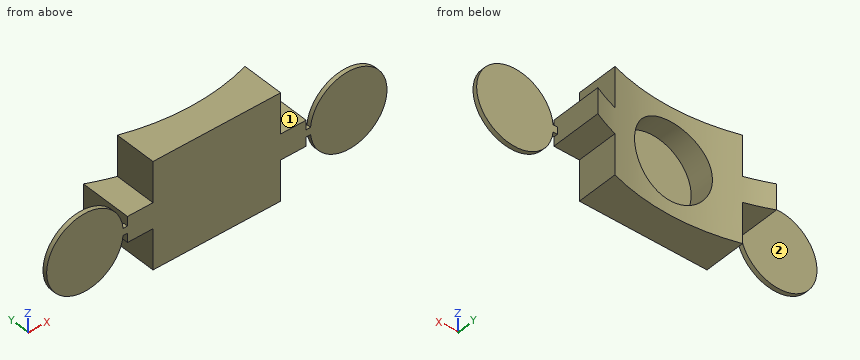
```python
from build123d import *

# Parameters (mm, degrees)
F1_DEPTH  = 12.5
F3_DEPTH  = 25
F4_R      = 9.15
F5_DEPTH  = 55
F6_R      = 9.05
F7_DEPTH  = 52.5
F9_DEPTH  = 3
F11_DEPTH = 57.501
F13_DEPTH = 1


with BuildPart() as f1:
    # F0 (on Top) → F1 (new body, symmetric)
    with BuildSketch(Plane.XY):
        with BuildLine():
            ThreePointArc((50, 0), (0, -50), (-50, 0))
            Line((-50, 0), (-55, 0))
            ThreePointArc((-55, 0), (0, -55), (55, 0))
            Line((55, 0), (50, 0))
        make_face()
    extrude(amount=F1_DEPTH, both=True)

    # F2 (on face) → F3 (join)
    with BuildSketch(Plane.XY.offset(12.5)):
        with BuildLine():
            ThreePointArc((55, 0), (0, -55), (-55, 0))
            Line((-55, 0), (-55, -57.5))
            Line((-55, -57.5), (0, -57.5))
            Line((0, -57.5), (55, -57.5))
            Line((55, -57.5), (55, 0))
        make_face()
    extrude(amount=-F3_DEPTH)

    # F4 (on Front) → F5 (cut)
    with BuildSketch(Plane.XZ):
        Circle(F4_R)
    extrude(amount=F5_DEPTH, mode=Mode.SUBTRACT)

    # F6 (on Right) → F7 (cut, symmetric)
    with BuildSketch(Plane.YZ):
        with Locations((-11, 0)):
            Circle(F6_R)
    extrude(amount=F7_DEPTH, both=True, mode=Mode.SUBTRACT)

    # F8 (on face) → F9 (join)
    with BuildSketch(Plane.XZ.offset(57.5)):
        with BuildLine():
            Line((55, -1.825145), (56.187007, -1.825145))
            ThreePointArc((56.187007, -1.825145), (73.996764, 0.241309), (56.101841, 1.350101))
            Line((56.101841, 1.350101), (55, 1.350101))
            Line((55, 1.350101), (55, -1.825145))
        make_face()
        with BuildLine():
            Line((-55, 0.589209), (-56.019308, 0.589209))
            ThreePointArc((-56.019308, 0.589209), (-73.999691, -0.074534), (-56.010781, -0.440385))
            Line((-56.010781, -0.440385), (-55, -0.440385))
            Line((-55, -0.440385), (-55, 0.589209))
        make_face()
        with BuildLine():
            Line((26.665892, -12.5), (26.665892, -13.538735))
            ThreePointArc((26.665892, -13.538735), (27.491135, -31.499996), (28.35176, -13.540396))
            Line((28.35176, -13.540396), (28.35176, -12.5))
            Line((28.35176, -12.5), (26.665892, -12.5))
        make_face()
        with BuildLine():
            Line((-28.294771, -12.5), (-28.294771, -13.535161))
            ThreePointArc((-28.294771, -13.535161), (-27.521055, -31.499975), (-26.663293, -13.538978))
            Line((-26.663293, -13.538978), (-26.663293, -12.5))
            Line((-26.663293, -12.5), (-28.294771, -12.5))
        make_face()
        with BuildLine():
            Line((-26.327094, 12.5), (-26.327094, 13.576756))
            ThreePointArc((-26.327094, 13.576756), (-27.667739, 31.498437), (-28.339533, 13.539242))
            Line((-28.339533, 13.539242), (-28.339533, 12.5))
            Line((-28.339533, 12.5), (-26.327094, 12.5))
        make_face()
        with BuildLine():
            Line((28.639116, 12.5), (28.639116, 13.572379))
            ThreePointArc((28.639116, 13.572379), (27.368028, 31.499032), (26.623167, 13.542815))
            Line((26.623167, 13.542815), (26.623167, 12.5))
            Line((26.623167, 12.5), (28.639116, 12.5))
        make_face()
    extrude(amount=-F9_DEPTH)

    # F10 (on face) → F11 (cut, through all)
    with BuildSketch(Plane.XZ.offset(57.5)):
        Polygon((-15, 3), (-15, 12.5), (-15, 43.200534), (-80.149591, 43.200534), (-80.149591, -41.894257), (-15, -41.894257), (-15, -12.5), (-15, -3), (-21, -3), (-21, 0), (-21, 3), align=None)
        Polygon((15, 42.100117), (15, 12.5), (15, 3), (21, 3), (21, 0), (21, -3), (15, -3), (15, -12.5), (15, -47.119375), (79.776369, -47.119375), (79.776369, 42.100117), align=None)
    extrude(amount=-F11_DEPTH, mode=Mode.SUBTRACT)

    # F12 (on face) → F13 (join)
    with BuildSketch(Plane.XZ.offset(57.5)):
        with BuildLine():
            Line((-21, 0.785101), (-22.034309, 0.785101))
            ThreePointArc((-22.034309, 0.785101), (-39.999944, 0.031742), (-22.04007, -0.848323))
            Line((-22.04007, -0.848323), (-21, -0.848323))
            Line((-21, -0.848323), (-21, 0.785101))
        make_face()
        with BuildLine():
            Line((21, -0.86237), (22.041411, -0.86237))
            ThreePointArc((22.041411, -0.86237), (39.99991, 0.040222), (22.034061, 0.782262))
            Line((22.034061, 0.782262), (21, 0.782262))
            Line((21, 0.782262), (21, -0.86237))
        make_face()
    extrude(amount=-F13_DEPTH)


solid = f1.part
```
Can you work these out from the model? Positions are in its coordinate system, mm. Face numbers are marked on the shaded views. A direction names the side the tool comes from. Round coordinates to 2 decimals unless told otherwise and drop trailing zeros. Order: outer loops, then holes, each group sorted by start corner. A loop starts at its lowest first (then second) coordinate and runs counter-clockwise, first axis right, second up.
(1) If we section it at C-C (y = -47): Please give me the cut outline in (x, z).
Results are:
outline: (-21, -3) - (-17.06, -3) - (-17.06, 3) - (-21, 3) - close; (17.06, -3) - (21, -3) - (21, 3) - (17.06, 3) - close
(2) On a 3-axis mill with a long thin cutter (end or side, diameter ignored), from which of +Z, -Z, +X, -X, +Y, -Y can I reach the whole of each face in a straight line? I mean the marked faces 1 and 2. Say none if no direction works.
Results are:
face 1: +Z, +Y, -Y
face 2: +Z, -Z, -X, +Y
(3) If we section it at B-B (y = -53.5): Please give me the cut outline in (x, z).
Results are:
outline: (-21, -3) - (-15, -3) - (-15, -12.5) - (15, -12.5) - (15, -3) - (21, -3) - (21, 3) - (15, 3) - (15, 12.5) - (-15, 12.5) - (-15, 3) - (-21, 3) - close; hole circle Ø18.3 at (0, 0)
(4) If we section it at A-A (z = 7.25): Please give me the cut outline in (x, y), plus the area to 3 significant figures.
Results are:
outline: (-36.33, -57.5) - (-25.67, -57.5) - (-25.67, -56.5) - (-36.33, -56.5) - close; (-15, -57.5) - (15, -57.5) - (15, -47.7) arc R50 cw to (5.58, -49.69) - (5.58, -55) - (-5.58, -55) - (-5.58, -49.69) arc R50 cw to (-15, -47.7) - close; (25.67, -57.5) - (36.33, -57.5) - (36.33, -56.5) - (25.67, -56.5) - close
area: 212 mm2
(5) I'm going to push flat-ended pins straight in: pin 1 (1 mm diameter, centred on x = 32, z = 8, fed in from +Y); pin 2 (1.8 mm diameter, centred on x = 17, y = -53.5, fed in from +Z); pin 3 (5 mm diameter, centred on y = -51.5, z = -7, fed in from -X). Where does each tip first touch, or does it pass through?
Results are:
pin 1: stops at y = -56.5
pin 2: stops at z = 3
pin 3: stops at x = -15
(6) If we section it at D-D (x = 0): Please give me the cut outline in (y, z).
Results are:
outline: (-57.5, -12.5) - (-50, -12.5) - (-50, -9.15) - (-55, -9.15) - (-55, 9.15) - (-50, 9.15) - (-50, 12.5) - (-57.5, 12.5) - close
(7) If I drill on L1, parallel to X at y = -52.9, z = 0; L2, parallel to Z at x = 0, y = -51.1; L3, parallel to Y at x = 5.5, z = 5, over which ranges is the centre line in solid material (lowest first)?
Results are:
L1: x = -21 to -9.15, 9.15 to 21
L2: z = -12.5 to -9.15, 9.15 to 12.5
L3: y = -57.5 to -55
